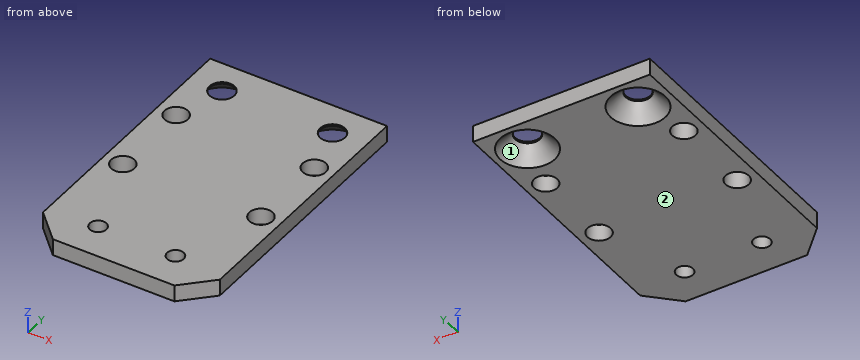
```python
from build123d import *

# Parameters (mm, degrees)
SKETCH_1_R      = 2.1
SKETCH_1_R_2    = 1.5
SKETCH_1_R_3    = 2.25
EXTRUDE_1_DEPTH = 3
CHAMFER_2_SIZE  = 2.7
CHAMFER_3_SIZE  = 2.7


with BuildPart() as part:
    # 草图1 → 拉伸1 (new body)
    with BuildSketch(Plane.XY):
        Polygon((-16, -21), (-11, -26), (11, -26), (16, -21), (16, 26), (-16, 26), align=None)
        with Locations((-12.5, 11)):
            Circle(SKETCH_1_R, mode=Mode.SUBTRACT)
        with Locations((12.5, 11)):
            Circle(SKETCH_1_R, mode=Mode.SUBTRACT)
        with Locations((12.5, -4)):
            Circle(SKETCH_1_R, mode=Mode.SUBTRACT)
        with Locations((-12.5, -4)):
            Circle(SKETCH_1_R, mode=Mode.SUBTRACT)
        with Locations((-7, -19.5)):
            Circle(SKETCH_1_R_2, mode=Mode.SUBTRACT)
        with Locations((7, -19.5)):
            Circle(SKETCH_1_R_2, mode=Mode.SUBTRACT)
        with Locations((10, 20)):
            Circle(SKETCH_1_R_3, mode=Mode.SUBTRACT)
        with Locations((-10, 20)):
            Circle(SKETCH_1_R_3, mode=Mode.SUBTRACT)
    extrude(amount=EXTRUDE_1_DEPTH)

    # 倒角2
    chamfer_2_edges = [part.edges().sort_by_distance(p)[0] for p in [
        (7.75, 20, 0),
    ]]
    chamfer(chamfer_2_edges, length=CHAMFER_2_SIZE)

    # 倒角3
    chamfer_3_edges = [part.edges().sort_by_distance(p)[0] for p in [
        (-12.25, 20, 0),
    ]]
    chamfer(chamfer_3_edges, length=CHAMFER_3_SIZE)


solid = part.part
```
Source: CAD feature listing. Evaluate the final solid. Frame: model axes, mm. Face numbers are marked on the shaded views. Coordinates: 2 decimals unless noted, no trailing zeros. Loops run counter-clockwise (first coordinate to the right, second up) from the corner with the lowest first, then second, coordinate; pieces in that order, holes last. Notation, with made-up numbers: (54, -35.5) -> (111, -35.5) arc R28 ccw to (111, -3.5) -> close; hole circle Ø8 at (-20.5, 10.5). An arc over 180 degrees is marked (long way). One line per item, written item: value. Start each with the question number.
Q1. Line query: line 1 along Y through (x, z) = (-10, 2.8); line 2 along Y through (x, z) = (7, 1); line 3 along X through (y, z) = (21.5, 1.25). Output: solid intervals per line, ascending.
Q2. Mould query, pull axis X, two halves, no side actions, for the marked faces 1 and 2. Classes: pulls with the +X half, pulls with the -X half, needs draft (parallel to the pull), parting line crosses it, or undercut.
Q3. Section query B-B, the plane z = 0.9. Give the number of separate pieces and of enclosed holes in the cut face, and give its area (3 significant figures).
Q4. Contact query for flat-ended pins moving along their axis: P1, Ø2.5, axis at x = 7, y = -19.5, coming from the -Z side; P2, Ø5, axis at x = 10, y = 20, coming from the -Z side. Output: stop coordinate, or through.
Q5. Section query C-C, the plane y = -19.5. Return the cut outline in (x, z), and give its area (3 significant figures).
Q6. Section query A-A, the plane y = 11. Return the cut outline in (x, z).
Results:
1. line 1: -26 to 17.75, 22.25 to 26
1. line 2: -26 to -21, -18 to 17.43, 22.57 to 26
1. line 3: -16 to -13.38, -6.62 to 6.62, 13.38 to 16
2. face 1: undercut
2. face 2: needs draft
3. separate pieces: 1
3. enclosed holes: 8
3. area: 1,470 mm^2
4. P1: through
4. P2: z = 2.45
5. outline: (-16, 0) -> (-8.5, 0) -> (-8.5, 3) -> (-16, 3) -> close; (-5.5, 0) -> (5.5, 0) -> (5.5, 3) -> (-5.5, 3) -> close; (8.5, 0) -> (16, 0) -> (16, 3) -> (8.5, 3) -> close
5. area: 78.0 mm^2
6. outline: (-16, 0) -> (-14.6, 0) -> (-14.6, 3) -> (-16, 3) -> close; (-10.4, 0) -> (10.4, 0) -> (10.4, 3) -> (-10.4, 3) -> close; (14.6, 0) -> (16, 0) -> (16, 3) -> (14.6, 3) -> close
